Check sheet for the drawn part. Datum: minimum x, y, z corner. Units: mm. A direction names the side the tool comes from. Coordinates: 2 decimals unless noted, no trailing zeros. Order: outer loops, then holes, each group sorted by start corner. A loop starts at its lowest first (then second) coordinate and runs counter-clockwise, first axis right, second up.
Q1. Thickness scan on line 1 (X direction, y = 7.25, z = 5.5); line 2 (Y direction, x = 19, z = 5.25); line 3 (Y direction, x = 14, z = 1.5). Record the ranges inside material, lowest first.
Q2. Cross-section at D-D, the plane x = 46.5. Record the boundary of the cut face in (y, z), and give its area (3 significant figures).
Q3. Set-up check for the marked faces 4 and 5: record each of +Z, -Z, +X, -X, +Y, -Y from which the full face is reachable in a straight line by a thin tool's end or side.
Q4. Cross-section at C-C, the plane x = 55. Record the boundary of the cut face in (y, z).
Q5. Draft check along X on the marked faces 1, 2 and 3. Enter one of: pulls with the +X half, pulls with the -X half, needs draft (parallel to the pull), parting line crosses it, or undercut.
Q6. Cross-section at A-A, the plane y = 4. Record the boundary of the cut face in (x, z), and give its area (3 significant figures).
Q7. Depth check by flat-ended pin: P1, Ø4, axis at y = 4.5, z = 3, coming from the -X side; P2, Ø1.5, axis at x = 35.5, z = 2, coming from the +Y side. Enter the tip coordinate at first touch or a pass-through.
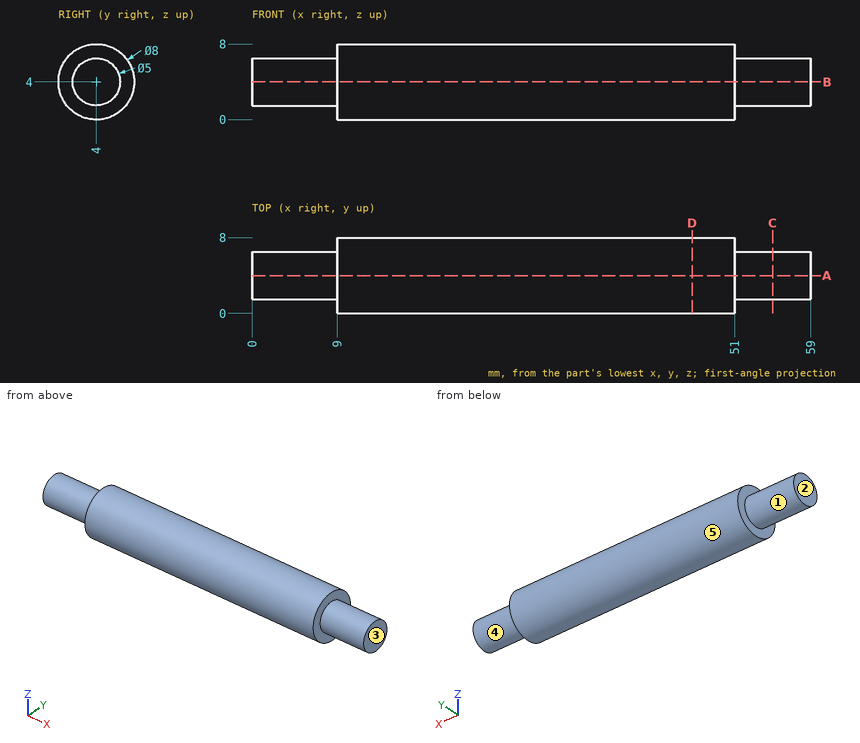
Check values:
1. line 1: x = 9 to 51
1. line 2: y = 0.2 to 7.8
1. line 3: y = 0.88 to 7.12
2. outline: circle Ø8 at (4, 4)
2. area: 50.3 mm2
3. face 4: +X
3. face 5: +X, -X
4. outline: circle Ø5 at (4, 4)
5. face 1: needs draft
5. face 2: pulls with the -X half
5. face 3: pulls with the +X half
6. outline: (0, 1.5) - (9, 1.5) - (9, 0) - (51, 0) - (51, 1.5) - (59, 1.5) - (59, 6.5) - (51, 6.5) - (51, 8) - (9, 8) - (9, 6.5) - (0, 6.5) - close
6. area: 421 mm2
7. P1: stops at x = 0
7. P2: stops at y = 7.8
